Autodesk Inventor part; units mm, degrees
ref_plane "YZ Plane" through (0, 0, 0) normal (1, 0, 0) x (0, 1, 0)
ref_plane "XZ Plane" through (0, 0, 0) normal (0, 1, 0) x (-1, 0, 0)
ref_plane "XY Plane" through (0, 0, 0) normal (0, 0, 1) x (1, 0, 0)
sketch "Sketch1" plane through (0, 0, 0) normal (0, 0, 1) x (1, 0, 0)
  line L0 (-18.6192, 22.6484) -> (22.0208, 22.6484)
  line L1 (22.0208, 22.6484) -> (22.0208, -17.9916)
  line L2 (22.0208, -17.9916) -> (-18.6192, -17.9916)
  line L3 (-18.6192, -17.9916) -> (-18.6192, 22.6484)
  dimension "d0" = 40.64
  dimension "d1" = 40.64
extrude "Extrusion1" add sketch "Sketch1" along normal blind 1.27
sketch "Sketch2" plane through (0, 0, 1.27) normal (0, 0, 1) x (1, 0, 0)
  line L0 (-18.6192, 22.6484) -> (22.0208, 22.6484)
  line L1 (-18.6192, -17.9916) -> (-18.6192, 22.6484)
  line L2 (-16.5872, 20.1084) -> (-12.7772, 20.1084)
  line L3 (-12.7772, 20.1084) -> (-12.7772, 18.8384)
  line L4 (-12.7772, 18.8384) -> (-16.5872, 18.8384)
  line L5 (-16.5872, 18.8384) -> (-16.5872, 20.1084)
  dimension "d4" = 2.54
  dimension "d5" = 1.27
  dimension "d6" = 2.032
  dimension "d7" = 3.81
extrude "Extrusion2" cut sketch "Sketch2" against normal through all
pattern_linear "Rectangular Pattern1" count 2 spacing 32.766 along (1, 0, 0) of "Extrusion2"
sketch "Sketch3" plane through (0, 0, 1.27) normal (0, 0, 1) x (1, 0, 0)
  line L0 (22.0208, 22.6484) -> (22.0208, -17.9916)
  line L1 (-18.6192, 22.6484) -> (22.0208, 22.6484)
  line L2 (-18.6192, -17.9916) -> (-18.6192, 22.6484)
  circle A0 centre (1.7008, 12.4884) radius 2.3876
  circle A1 centre (8.0508, 12.4884) radius 1.27
  circle A2 centre (1.7008, 12.4884) radius 20.32 construction
  dimension "d16" = 2.54
  dimension "d17" = 4.7752
  dimension "d18" = 6.35
  dimension "d19" = 10.16
extrude "Extrusion3" cut sketch "Sketch3" against normal through all
pattern_linear "Rectangular Pattern2" count 3 spacing 10.16 along (0, -1, 0) of "Extrusion3"
sketch "Sketch4" plane through (0, 0, 1.27) normal (0, 0, 1) x (1, 0, 0)
  line L0 (-18.6192, -17.9916) -> (-18.6192, 22.6484)
  line L1 (22.0208, -17.9916) -> (-18.6192, -17.9916)
  line L2 (-12.2692, -15.4516) -> (-8.4592, -15.4516)
  line L3 (-8.4592, -15.4516) -> (-8.4592, -14.1816)
  line L4 (-8.4592, -14.1816) -> (-12.2692, -14.1816)
  line L5 (-12.2692, -14.1816) -> (-12.2692, -15.4516)
  dimension "d25" = 3.81
  dimension "d26" = 1.27
  dimension "d27" = 2.54
  dimension "d28" = 6.35
extrude "Extrusion4" cut sketch "Sketch4" against normal through all
pattern_linear "Rectangular Pattern3" count 2 spacing 24.13 along (1, 0, 0) of "Extrusion4"
properties part number "fishpaper"
The listing builds one solid part. Answer for the finished solid, in the listing's coordinates (mm). A direction names the side the tool comes from. Round coordinates to 2 decimals unless told otherwise and drop trailing zeros. Order: outer loops, then holes, each group sorted by start corner. A loop starts at its lowest first (then second) coordinate and runs counter-clockwise, first axis right, second up. Notation, with made-up numbers: (76, -39) -> (99, -39) arc R15 ccw to (99, -30) -> close; hole circle Ø1 at (-34, -18.75). An arc over 180 degrees is marked (long way). Answer as CSV lines item,"result". Start each with the question number.
(1) Find the intervals of material crossed by probe 1 along Y at (x, z) = (8, 1.2); probe 2 along X at (y, z) = (-15, 0.65); probe 3 along Y at (x, z) = (19, 1), in increasing order. Write a range as from..to.
(2) The part is cut by section B-B (z = 0.5). Count the separate pieces of the cut face and the enclosed holes in it, then the cut area to 3 significant figures.
(3) For a pull along X with two mould halves and no side action, classify faces 1 (the face through (1, 7, 1.27)), 2 (the face through (14, -14.182, 1)) as +X half, -X half, draft (parallel to the pull), parting line (faces both ways), or undercut.
(4) A tool of negligible diameter and unlimited length cuts with its end or side. For faces 3 (the face through (2, -17.992, 1)), 4 (the face through (-16.587, 19, 1)), from which of +Z, -Z, +X, -X, +Y, -Y can it reach the whole face along a straight path? Write none if from no direction.
(5) The part is cut by section A-A (y = 0.5). Determine the outline of the cut face in (x, z).
Evaluation:
1,probe 1,"-17.99..-9.1, -6.56..1.06, 3.6..11.22, 13.76..22.65"
1,probe 2,"-18.62..-12.27, -8.46..11.86, 15.67..22.02"
1,probe 3,"-17.99..18.84, 20.11..22.65"
2,separate pieces,"1"
2,enclosed holes,"10"
2,area,"1,560 mm²"
3,face 1,"draft"
3,face 2,"undercut"
4,face 3,"+Z, -Z, +X, -X, -Y"
4,face 4,"+Z, -Z"
5,outline,"(-18.62, 0) -> (0.17, 0) -> (0.17, 1.27) -> (-18.62, 1.27) -> close; (3.24, 0) -> (22.02, 0) -> (22.02, 1.27) -> (3.24, 1.27) -> close"
